```python
from build123d import *

# Parameters (mm, degrees)
EXTRUSION1_DEPTH        = 1
ESQUISSE14_W            = 38
ESQUISSE14_H            = 1.021269028
ESQUISSE14_H_2          = 0.92452696
EXTRUSION2_DEPTH        = 17
CONG_3_R                = 3
ESQUISSE20_R            = 1.551729924
ESQUISSE20_R_2          = 1.5
ENL_V_MAT_EXTRU_7_DEPTH = 46


with BuildPart() as part:
    # Esquisse1 → Extrusion1 (new body)
    with BuildSketch(Plane.XY):
        Polygon((-30.989172535, 10.739018032), (-30.989172535, -22.260981968), (-37.989172535, -22.260981968), (-37.989172535, -28.260981968), (-53.989172535, -28.260981968), (-53.989172535, -22.260981968), (-68.989172535, -22.260981968), (-68.989172535, 10.739018032), (-53.989172535, 10.739018032), (-53.989172535, 16.739018032), (-37.989172535, 16.739018032), (-37.989172535, 10.739018032), align=None)
    extrude(amount=EXTRUSION1_DEPTH)

    # Esquisse14 → Extrusion2 (add)
    with BuildSketch(Plane.XY.offset(1)):
        with Locations((-49.989172535, 10.228383518)):
            Rectangle(ESQUISSE14_W, ESQUISSE14_H)
        with Locations((-49.989172535, -21.798718488)):
            Rectangle(ESQUISSE14_W, ESQUISSE14_H_2)
    extrude(amount=EXTRUSION2_DEPTH)

    # Congé3
    cong_3_edges = [part.edges().sort_by_distance(p)[0] for p in [
        (-68.989172535, -21.798718488, 18),
        (-30.989172535, -21.798718488, 18),
        (-30.989172535, 10.228383518, 18),
        (-68.989172535, 10.228383518, 18),
    ]]
    fillet(cong_3_edges, radius=CONG_3_R)

    # Esquisse20 → Enlèv. mat.-Extru.7 (cut)
    with BuildSketch(Plane(origin=(0, 10.739018032, 0), x_dir=(-1, 0, 0), z_dir=(0, 1, 0))):
        with Locations((109.664285954, 11.585691392)):
            Circle(ESQUISSE20_R)
        with Locations(Location((58.989172535, 11, 0), (0, 0, 90))):
            Circle(ESQUISSE20_R_2)
    extrude(amount=-ENL_V_MAT_EXTRU_7_DEPTH, mode=Mode.SUBTRACT)


solid = part.part
```
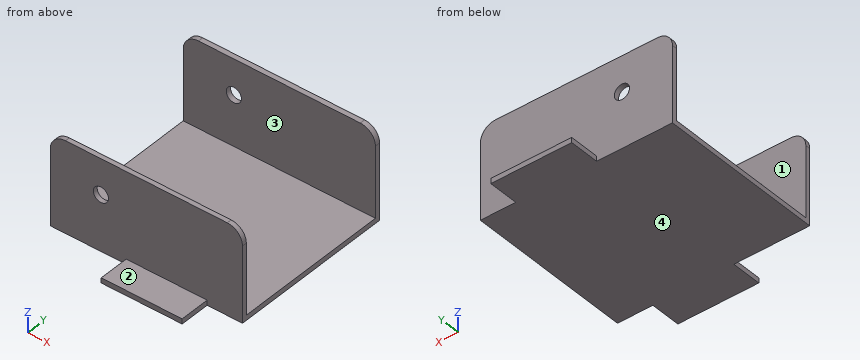
Can you work these out from the model? Positions are in its coordinate system, mm. Face numbers are marked on the shaded views. A direction names the side the tool comes from. Coordinates: 2 decimals unless noted, no trailing zeros. Write each loop counter-clockwise with the first axis right and the second up, starting at its lowest first coordinate (ties: lowest second). Pieces come first, ordered by that corner, then holes. Notation, with made-up numbers: (37, 21) - (52, 21) arc R11 cw to (52, 30) - close; hole circle Ø8 at (51.25, -18.5). An arc over 180 degrees is marked (long way). Return JSON: item names as keys, results as strings.
Q1. I'm going to push flat-ended pins straight in: pin 1 Ø3 at (x, y) = (-35.5, -12) entering from +Z; pin 2 Ø5 at (x, z) = (-55, 7) entering from -Y; pin 3 Ø1.1 at (y, z) = (-25, 0.5) entering from -X; pin 4 Ø2.5 at (x, z) = (-58.99, 11) entering from +Y. Where does each tip first touch, or does it pass through?
Computed values:
{"pin 1": "stops at z = 1", "pin 2": "stops at y = -22.26", "pin 3": "stops at x = -53.99", "pin 4": "passes through"}
Q2. If we section it at A-A (z = 8): Please give me the cut outline in (x, y).
Computed values:
{"outline": "(-68.99, -22.26) - (-30.99, -22.26) - (-30.99, -21.34) - (-68.99, -21.34) - close; (-68.99, 9.72) - (-30.99, 9.72) - (-30.99, 10.74) - (-68.99, 10.74) - close"}
Q3. Please list where these lines run through material, in increasing order: L1, parallel to Y at x = -44, z = 5.25; L2, parallel to X at y = 10.35, z = 11; L3, parallel to Z at x = -35.5, y = -8. Write a range as from..to.
Computed values:
{"L1": "y = -22.26..-21.34, 9.72..10.74", "L2": "x = -68.99..-60.49, -57.49..-30.99", "L3": "z = 0..1"}
Q4. If we section it at D-D (z = 15.75): Please give me the cut outline in (x, y).
Computed values:
{"outline": "(-68.89, -22.26) - (-31.08, -22.26) - (-31.08, -21.34) - (-68.89, -21.34) - close; (-68.89, 9.72) - (-31.08, 9.72) - (-31.08, 10.74) - (-68.89, 10.74) - close"}
Q5. If we section it at B-B (x = -61): Please give me the cut outline in (y, z), then the cut area to 3 significant figures.
Computed values:
{"outline": "(-22.26, 0) - (10.74, 0) - (10.74, 18) - (9.72, 18) - (9.72, 1) - (-21.34, 1) - (-21.34, 18) - (-22.26, 18) - close", "area": "66.1 mm2"}
Q6. If we section it at C-C (z = 11): Please give me the cut outline in (x, y).
Computed values:
{"outline": "(-68.99, -22.26) - (-60.49, -22.26) - (-60.49, -21.34) - (-68.99, -21.34) - close; (-68.99, 9.72) - (-60.49, 9.72) - (-60.49, 10.74) - (-68.99, 10.74) - close; (-57.49, -22.26) - (-30.99, -22.26) - (-30.99, -21.34) - (-57.49, -21.34) - close; (-57.49, 9.72) - (-30.99, 9.72) - (-30.99, 10.74) - (-57.49, 10.74) - close"}
Q7. On a 3-axis mill with a long thin cutter (end or side, diameter ignored), from which of +Z, -Z, +X, -X, +Y, -Y can I reach the whole of each face in a straight line? I mean the marked faces 3 and 4. Say none if no direction works.
Computed values:
{"face 3": "+Z, +X, -X", "face 4": "-Z, +X, -X, +Y, -Y"}
Q8. Thinking about a two-plate mould opening in Y: for the marked faces 1 and 2, which applies, +Y half, -Y half, draft (parallel to the pull), parting line (faces both ways), or undercut?
Computed values:
{"face 1": "undercut", "face 2": "draft"}
